Check sheet for the modelled part. Datum: model origin and axes. Units: mm. A direction names the side the tool comes from. Give positions to 0.01 mm unless a question says otherwise; leave off trailing zeros. Write each loop counter-clockwise with the first axis right and the second up, starting at its lowest first coordinate (ties: lowest second). Pieces come first, ordered by that corner, then holes. Notation, with made-up numbers: (44, -18) -> (82, -18) arc R33 ccw to (82, 20) -> close; hole circle Ø5 at (77, -30.5). An arc over 180 degrees is marked (long way). Return JSON: item names as keys, results as strings.
from build123d import *

# Parameters (mm, degrees)
RESSALTO_EXTRUS_O1_DEPTH           = 38
FILETE1_R                          = 4
CASCA1_T                           = -1.5
CORTE_EXTRUS_O1_DEPTH              = 50
ESBO_O3_R                          = 2
ESBO_O3_R_2                        = 1
RESSALTO_EXTRUS_O2_DEPTH           = 5
RESSALTO_EXTRUS_O2_DRAFT           = 2
RESSALTO_EXTRUS_O2_PROFILE_2_DEPTH = 5
RESSALTO_EXTRUS_O2_PROFILE_2_DRAFT = 2
RESSALTO_EXTRUS_O2_PROFILE_3_DEPTH = 5
RESSALTO_EXTRUS_O2_PROFILE_3_DRAFT = 2
RESSALTO_EXTRUS_O2_PROFILE_4_DEPTH = 5
RESSALTO_EXTRUS_O2_PROFILE_4_DRAFT = 2
RESSALTO_EXTRUS_O3_DEPTH           = 1
RESSALTO_EXTRUS_O4_DEPTH           = 5.5
ESBO_O6_R                          = 10
CORTE_EXTRUS_O2_DEPTH              = 75.848179671


with BuildPart() as part:
    # Esboço1 → Ressalto-extrusão1 (new body)
    with BuildSketch(Plane(origin=(0, 0, 0), x_dir=(1, 0, 0), z_dir=(0, 1, 0))):
        with BuildLine():
            Line((-44.5, 35), (44.5, 35))
            ThreePointArc((44.5, 35), (47.328427125, 33.828427125), (48.5, 31))
            Line((48.5, 31), (48.5, -31))
            ThreePointArc((48.5, -31), (47.328427125, -33.828427125), (44.5, -35))
            Line((44.5, -35), (-44.5, -35))
            ThreePointArc((-44.5, -35), (-47.328427125, -33.828427125), (-48.5, -31))
            Line((-48.5, -31), (-48.5, 31))
            ThreePointArc((-48.5, 31), (-47.328427125, 33.828427125), (-44.5, 35))
        make_face()
    extrude(amount=-RESSALTO_EXTRUS_O1_DEPTH)

    # Filete1
    filete1_edges = [part.edges().sort_by_distance(p)[0] for p in [
        (48.5, 0, 0),
        (47.328427125, 0, 33.828427125),
        (0, 0, 35),
        (-47.328427125, 0, 33.828427125),
        (-48.5, 0, 0),
        (-47.328427125, 0, -33.828427125),
        (0, 0, -35),
        (47.328427125, 0, -33.828427125),
    ]]
    fillet(filete1_edges, radius=FILETE1_R)

    # Casca1
    casca1_openings = [part.faces().sort_by_distance(p)[0] for p in [
        (0, -38, 0),
    ]]
    offset(amount=CASCA1_T, openings=casca1_openings, kind=Kind.INTERSECTION)

    # Esboço2 → Corte-extrusão1 (cut, symmetric)
    with BuildSketch(Plane(origin=(0, 0, 0), x_dir=(0, 0, -1), z_dir=(1, 0, 0))):
        with BuildLine():
            Line((-21.110742301, -6), (21.110742301, -6))
            ThreePointArc((21.110742301, -6), (23.68189274, -6.935822228), (25.049973313, -9.305407289))
            Line((25.049973313, -9.305407289), (31, -43.049685465))
            Line((31, -43.049685465), (-31, -43.049685465))
            Line((-31, -43.049685465), (-25.049973313, -9.305407289))
            ThreePointArc((-25.049973313, -9.305407289), (-23.68189274, -6.935822228), (-21.110742301, -6))
        make_face()
    extrude(amount=CORTE_EXTRUS_O1_DEPTH, both=True, mode=Mode.SUBTRACT)


with BuildPart() as ressalto_extrus_o2_tool:
    # Esboço3 → Ressalto-extrusão2 (with draft: the straight prism first)
    with BuildSketch(Plane.XZ.offset(1.5)):
        with Locations((-28, 15)):
            Circle(ESBO_O3_R)
        with Locations((-28, 15)):
            Circle(ESBO_O3_R_2, mode=Mode.SUBTRACT)
    extrude(amount=RESSALTO_EXTRUS_O2_DEPTH)
    # Ressalto-extrusão2: the draft: its side faces are tilted about the plane it starts from
    ressalto_extrus_o2_sides = [ressalto_extrus_o2_tool.faces().sort_by_distance(p)[0] for p in [
        (-30, -4, 15),
        (-29, -4, 15),
    ]]
    draft(ressalto_extrus_o2_sides, Plane.XZ.offset(1.5), RESSALTO_EXTRUS_O2_DRAFT)


with BuildPart() as part_1:
    add(part.part)

    # Ressalto-extrusão2: add ressalto_extrus_o2_tool
    add(ressalto_extrus_o2_tool.part)


with BuildPart() as ressalto_extrus_o2_profile_2_tool:
    # Esboço3 → Ressalto-extrusão2 profile 2 (with draft: the straight prism first)
    with BuildSketch(Plane.XZ.offset(1.5)):
        with Locations((28, 15)):
            Circle(ESBO_O3_R)
        with Locations((28, 15)):
            Circle(ESBO_O3_R_2, mode=Mode.SUBTRACT)
    extrude(amount=RESSALTO_EXTRUS_O2_PROFILE_2_DEPTH)
    # Ressalto-extrusão2 profile 2: the draft: its side faces are tilted about the plane it starts from
    ressalto_extrus_o2_profile_2_sides = [ressalto_extrus_o2_profile_2_tool.faces().sort_by_distance(p)[0] for p in [
        (26, -4, 15),
        (27, -4, 15),
    ]]
    draft(ressalto_extrus_o2_profile_2_sides, Plane.XZ.offset(1.5), RESSALTO_EXTRUS_O2_PROFILE_2_DRAFT)


with BuildPart() as part_2:
    add(part_1.part)

    # Ressalto-extrusão2 profile 2: add ressalto_extrus_o2_profile_2_tool
    add(ressalto_extrus_o2_profile_2_tool.part)


with BuildPart() as ressalto_extrus_o2_profile_3_tool:
    # Esboço3 → Ressalto-extrusão2 profile 3 (with draft: the straight prism first)
    with BuildSketch(Plane.XZ.offset(1.5)):
        with Locations((28, -15)):
            Circle(ESBO_O3_R)
        with Locations((28, -15)):
            Circle(ESBO_O3_R_2, mode=Mode.SUBTRACT)
    extrude(amount=RESSALTO_EXTRUS_O2_PROFILE_3_DEPTH)
    # Ressalto-extrusão2 profile 3: the draft: its side faces are tilted about the plane it starts from
    ressalto_extrus_o2_profile_3_sides = [ressalto_extrus_o2_profile_3_tool.faces().sort_by_distance(p)[0] for p in [
        (26, -4, -15),
        (27, -4, -15),
    ]]
    draft(ressalto_extrus_o2_profile_3_sides, Plane.XZ.offset(1.5), RESSALTO_EXTRUS_O2_PROFILE_3_DRAFT)


with BuildPart() as part_3:
    add(part_2.part)

    # Ressalto-extrusão2 profile 3: add ressalto_extrus_o2_profile_3_tool
    add(ressalto_extrus_o2_profile_3_tool.part)


with BuildPart() as ressalto_extrus_o2_profile_4_tool:
    # Esboço3 → Ressalto-extrusão2 profile 4 (with draft: the straight prism first)
    with BuildSketch(Plane.XZ.offset(1.5)):
        with Locations((-28, -15)):
            Circle(ESBO_O3_R)
        with Locations((-28, -15)):
            Circle(ESBO_O3_R_2, mode=Mode.SUBTRACT)
    extrude(amount=RESSALTO_EXTRUS_O2_PROFILE_4_DEPTH)
    # Ressalto-extrusão2 profile 4: the draft: its side faces are tilted about the plane it starts from
    ressalto_extrus_o2_profile_4_sides = [ressalto_extrus_o2_profile_4_tool.faces().sort_by_distance(p)[0] for p in [
        (-30, -4, -15),
        (-29, -4, -15),
    ]]
    draft(ressalto_extrus_o2_profile_4_sides, Plane.XZ.offset(1.5), RESSALTO_EXTRUS_O2_PROFILE_4_DRAFT)


with BuildPart() as part_4:
    add(part_3.part)

    # Ressalto-extrusão2 profile 4: add ressalto_extrus_o2_profile_4_tool
    add(ressalto_extrus_o2_profile_4_tool.part)

    # Esboço4 → Ressalto-extrusão3 (add)
    with BuildSketch(Plane.XY.offset(35)):
        with BuildLine():
            Line((-9, -38), (9, -38))
            Line((9, -38), (9, -44))
            ThreePointArc((9, -44), (8.707106781, -44.707106781), (8, -45))
            Line((8, -45), (-8, -45))
            ThreePointArc((-8, -45), (-8.707106781, -44.707106781), (-9, -44))
            Line((-9, -44), (-9, -38))
        make_face()
    ressalto_extrus_o3 = extrude(amount=-RESSALTO_EXTRUS_O3_DEPTH)

    # Esboço5 → Ressalto-extrusão4 (add, symmetric)
    with BuildSketch(Plane(origin=(0, 0, 0), x_dir=(0, 0, -1), z_dir=(1, 0, 0))):
        Polygon((-34, -40), (-32.5, -40), (-32.5, -40.5), (-34, -42), align=None)
    ressalto_extrus_o4 = extrude(amount=RESSALTO_EXTRUS_O4_DEPTH, both=True)

    # Espelhar1: Ressalto-extrusão3, Ressalto-extrusão4 across plane
    add(ressalto_extrus_o3.mirror(Plane.XY))
    add(ressalto_extrus_o4.mirror(Plane.XY))

    # Esboço6 → Corte-extrusão2 (cut, through all)
    with BuildSketch(Plane(origin=(0, 0, 0), x_dir=(1, 0, 0), z_dir=(0, 1, 0))):
        with Locations(Location((-5, 0.5, 0), (0, 0, 270))):
            Circle(ESBO_O6_R)
    extrude(amount=-CORTE_EXTRUS_O2_DEPTH, mode=Mode.SUBTRACT)


solid = part_4.part
(1) Depth check by flat-ended pin: pin 1 Ø1.2 at (y, z) = (-41, 33) entering from -X; pin 2 Ø0.8 at (y, z) = (-40.5, -34.5) entering from +X; pin 3 Ø1.8 at (x, z) = (29, 14) entering from -Y. Enter the tip coordinate at first touch or a pass-through.
Reply:
{"pin 1": "x = -5.5", "pin 2": "x = 9", "pin 3": "y = -6.5"}
(2) Cross-section at A-A on z = -0.5. Enter the section's corners in (x, y), then the cut area to 3 significant figures.
Reply:
{"outline": "(-48.5, -6) -> (-47, -6) -> (-47, -4) arc R2.5 cw to (-44.5, -1.5) -> (-15, -1.5) -> (-15, 0) -> (-44.5, 0) arc R4 ccw to (-48.5, -4) -> close; (5, -1.5) -> (44.5, -1.5) arc R2.5 cw to (47, -4) -> (47, -6) -> (48.5, -6) -> (48.5, -4) arc R4 ccw to (44.5, 0) -> (5, 0) -> close", "area": "125 mm^2"}
(3) Release check for a two-part mould opening along Z. For faces 4 (the conical face through (-29.085, -3.965, -14.952)), 5 (the cylindrical face through (-0.623, -1.203, 33.859)) record: pulls with the +Z half, pulls with the -Z half, needs draft (parallel to the pull), parting line crosses it, or undercut.
Reply:
{"face 4": "undercut", "face 5": "pulls with the +Z half"}
(4) Cross-section at C-C on x = -20. Enter the section's corners in (y, z).
Reply:
{"outline": "(-38, -35) -> (-4, -35) arc R4 ccw to (0, -31) -> (0, 31) arc R4 ccw to (-4, 35) -> (-38, 35) -> (-38, 33.5) -> (-4, 33.5) arc R2.5 cw to (-1.5, 31) -> (-1.5, -31) arc R2.5 cw to (-4, -33.5) -> (-38, -33.5) -> close"}
(5) Thickness scan on L1, parallel to Z at x = 18, y = -31.5; L2, parallel to X at y = -27.5, z = -31; L3, parallel to Y at x = -21, z = -16. Record the ranges inside material, lowest first.
Reply:
{"L1": "-35 to -33.5, 33.5 to 35", "L2": "-48.5 to -47, 47 to 48.5", "L3": "-1.5 to 0"}
(6) Cross-section at D-D on x = 2. Enter the section's corners in (y, z), then the cut area to 3 significant figures.
Reply:
{"outline": "(-45, -35) -> (-4, -35) arc R4 ccw to (0, -31) -> (0, -7.64) -> (-1.5, -7.64) -> (-1.5, -31) arc R2.5 cw to (-4, -33.5) -> (-38, -33.5) -> (-38, -34) -> (-40, -34) -> (-40, -32.5) -> (-40.5, -32.5) -> (-42, -34) -> (-45, -34) -> close; (-45, 34) -> (-42, 34) -> (-40.5, 32.5) -> (-40, 32.5) -> (-40, 34) -> (-38, 34) -> (-38, 33.5) -> (-4, 33.5) arc R2.5 cw to (-1.5, 31) -> (-1.5, 6.64) -> (0, 6.64) -> (0, 31) arc R4 ccw to (-4, 35) -> (-45, 35) -> close", "area": "207 mm^2"}
(7) Cross-section at B-B on y = -20. Enter the section's corners in (x, z), then the cut area to 3 significant figures.
Reply:
{"outline": "(-48.5, -31) arc R4 ccw to (-44.5, -35) -> (44.5, -35) arc R4 ccw to (48.5, -31) -> (48.5, -26.94) -> (47, -26.94) -> (47, -31) arc R2.5 cw to (44.5, -33.5) -> (-44.5, -33.5) arc R2.5 cw to (-47, -31) -> (-47, -26.94) -> (-48.5, -26.94) -> close; (-48.5, 26.94) -> (-47, 26.94) -> (-47, 31) arc R2.5 cw to (-44.5, 33.5) -> (44.5, 33.5) arc R2.5 cw to (47, 31) -> (47, 26.94) -> (48.5, 26.94) -> (48.5, 31) arc R4 ccw to (44.5, 35) -> (-44.5, 35) arc R4 ccw to (-48.5, 31) -> close", "area": "322 mm^2"}
(8) Set-up check for faces 1 (the cylindrical face through (-14.76, -0.74, -2.67)), 2 (the cylindrical face through (-47.74, -6.96, 23.71)), 3 (the cylindrical face through (-46, -21, -33)): record each of +Z, -Z, +X, -X, +Y, -Y from which the full face is reachable in a straight line by a thin tool's end or side.
Reply:
{"face 1": "+Y, -Y", "face 2": "+X, -X, -Y", "face 3": "-Y"}
